The model under review builds one solid part; all positions refer to its coordinate system, in mm. A direction names the side the tool comes from. Coordinates: 2 decimals unless noted, no trailing zeros. Loops run counter-clockwise (first coordinate to the right, second up) from the corner with the lowest first, then second, coordinate; pieces in that order, holes last. Notation, with made-up numbers: M 52.25,75 L 64.25,75 A13 cw 64.25,79 Z; hole C -31,-33.5 d8. An arc over 180 degrees is marked long. Return JSON: item names as keys, results as strings.
```python
from build123d import *

# Parameters (mm, degrees)
F0_R     = 200
F0_R_2   = 198
F1_DEPTH = 655
F0_R_3   = 240
F0_R_4   = 6
F2_DEPTH = 5
F4_R     = 5
F5_SIZE  = 1
F6_SIZE  = 1
F8_D     = 300
F8_DEPTH = 240.001


# Not quite as in the source:
# - a fillet or chamfer that OpenCascade refuses, or shapes differently, is made with other operations: its cross-section is extruded or revolved along the edge and cut away or added
# - a feature names something its author has since deleted; it is built from what else it names


with BuildPart() as f1:
    # F0 (on Front) → F1 (new body)
    with BuildSketch(Plane.XZ):
        Circle(F0_R)
        Circle(F0_R_2, mode=Mode.SUBTRACT)
    extrude(amount=F1_DEPTH)

    # F0 (on Front) → F2 (join)
    with BuildSketch(Plane.XZ):
        Circle(F0_R_3)
        with Locations((-148.3494010818, -162.4575489125)):
            Circle(F0_R_4, mode=Mode.SUBTRACT)
        with Locations((-24.5270352061, -218.6285080771)):
            Circle(F0_R_4, mode=Mode.SUBTRACT)
        with Locations((-215.5073379549, -44.2333277925)):
            Circle(F0_R_4, mode=Mode.SUBTRACT)
        with Locations((108.663824475, -191.2908080658)):
            Circle(F0_R_4, mode=Mode.SUBTRACT)
        with Locations((200.3487965542, -90.8865211088)):
            Circle(F0_R_4, mode=Mode.SUBTRACT)
        with Locations((-200.0304758549, 90.5413627625)):
            Circle(F0_R_4, mode=Mode.SUBTRACT)
        with Locations((-108.663824475, 191.2908080658)):
            Circle(F0_R_4, mode=Mode.SUBTRACT)
        Circle(F0_R, mode=Mode.SUBTRACT)
        with Locations((215.5073379549, 44.2333277925)):
            Circle(F0_R_4, mode=Mode.SUBTRACT)
        with Locations((23.8151364028, 219.3368971348)):
            Circle(F0_R_4, mode=Mode.SUBTRACT)
        with Locations((148.3494010818, 162.4575489125)):
            Circle(F0_R_4, mode=Mode.SUBTRACT)
        Circle(F0_R)
        Circle(F0_R_2, mode=Mode.SUBTRACT)
    extrude(amount=-F2_DEPTH)

    # F3: fillet of radius 5 on 1 edges, made by hand

    # F3_s1 → F3_t2 (revolve, cut)
    with BuildSketch(Plane.XY):
        with BuildLine():
            ThreePointArc((198, 0), (199.4644660941, 3.5355339059), (203, 5))
            Line((203, 5), (198, 5))
            Line((198, 5), (198, 0))
        make_face()
    revolve(axis=Axis((0, 5, 0), (0, -1, 0)), mode=Mode.SUBTRACT)

    # F4
    f4_edges = [f1.edges().sort_by_distance(p)[0] for p in [
        (-200, 0, 0),
    ]]
    fillet(f4_edges, radius=F4_R)

    # F5
    f5_edges = [f1.edges().sort_by_distance(p)[0] for p in [
        (-205, 0, 0),
        (-240, 0, 0),
        (-154.349401, 0, -162.457549),
        (-30.527035, 0, -218.628508),
        (-221.507338, 0, -44.233328),
        (102.663824, 0, -191.290808),
        (194.348797, 0, -90.886521),
        (-206.030476, 0, 90.541363),
        (-114.663824, 0, 191.290808),
        (209.507338, 0, 44.233328),
        (17.815136, 0, 219.336897),
        (142.349401, 0, 162.457549),
    ]]
    chamfer(f5_edges, length=F5_SIZE)

    # F6
    f6_edges = [f1.edges().sort_by_distance(p)[0] for p in [
        (-240, 5, 0),
        (-154.349401, 5, -162.457549),
        (-30.527035, 5, -218.628508),
        (-221.507338, 5, -44.233328),
        (102.663824, 5, -191.290808),
        (-203, 5, 0),
        (194.348797, 5, -90.886521),
        (-206.030476, 5, 90.541363),
        (-114.663824, 5, 191.290808),
        (209.507338, 5, 44.233328),
        (17.815136, 5, 219.336897),
        (142.349401, 5, 162.457549),
    ]]
    chamfer(f6_edges, length=F6_SIZE)

    # F8 (through all, one way)
    with BuildSketch(Plane(origin=(0, 0, 0), x_dir=(1, 0, 0), z_dir=(0, 0, -1))):
        with Locations((0, 178.1619042158)):
            Circle(F8_D / 2)
    extrude(amount=-F8_DEPTH, mode=Mode.SUBTRACT)


solid = f1.part
```
1. The part is to be moulded in two halves that separate along Y. For faces 3 (the face through (104.52, -285.75, 169.7)), 4 (the face through (-239.77, 2.48, 10.55)), 5 (the face through (-54, 5, 196)), 6 (the face through (194, 0, 72)), say which applies: released by +Y, released by -Y, zero draft, split by the parting line, or undercut.
Check values:
{"face 3": "undercut", "face 4": "zero draft", "face 5": "released by +Y", "face 6": "released by -Y"}
2. Add section B-B on z = 0. Give the boundary of the cut face in (x, y).
Check values:
{"outline": "M -240,1 L -239,0 L -205,0 A5 cw -200,-5 L -200,-655 L -198,-655 L -198,0 A5 ccw -203,5 L -239,5 L -240,4 Z; M 198,-655 L 200,-655 L 200,-5 A5 cw 205,0 L 239,0 L 240,1 L 240,4 L 239,5 L 203,5 A5 ccw 198,0 Z"}
3. Add section C-C on y = -349. Give the boundary of the cut face in (x, z).
Check values:
{"outline": "C 0,0 d400; hole C 0,0 d396"}
4. Insertion check: pin 1 Ø11 at (x, z) = (108.66, -191.29) entering from -Y; pin 2 Ø19 at (x, z) = (-215.51, -44.23) entering from -Y; pin 3 Ø8 at (x, y) = (94, -250) entering from +Z; pin 4 Ø1 at (y, z) = (-350, -75) entering from -X. Each pin has a flat end and moves straight along its axis. Give the tip position at first contact, or say it passes through.
Check values:
{"pin 1": "through", "pin 2": "y = 0", "pin 3": "z = -172.05", "pin 4": "x = -185.61"}
5. Add section D-D on y = -189. Give the boundary of the cut face in (x, z).
Check values:
{"outline": "M -149.61,129.7 L -149.61,132.73 A200 ccw long 149.61,132.73 L 149.61,129.7 A198 cw long Z"}
6. Machinability: for faces 1 (the face through (-194, -655, 45)), 2 (the face through (-43.356, -325.45, -195.244)), which of the approach directions +Z, -Z, +X, -X, +Y, -Y give a long, thin tool a straight path to every point of the face, cutting with its end or side? Answer none if there is none.
Check values:
{"face 1": "+Z, -Z, +X, -X, -Y", "face 2": "-Y"}
7. To check wall thickness, follow line 1 (X direction, y = -199, z = -3); line 2 (Z direction, x = 8.5, y = -376); line 3 (Y direction, x = -133.5, z = -176). State the ranges of each line that lie inside material, in increasing order.
Check values:
{"line 1": "-199.98 to -197.98, 197.98 to 199.98", "line 2": "-199.82 to -197.82, 197.82 to 199.82", "line 3": "0 to 5"}
8. Add section A-A on x = 0. Give the boundary of the cut face in (y, z), plus the area to 3 significant figures.
Check values:
{"outline": "M -655,-200 L -5,-200 A5 cw 0,-205 L 0,-239 L 1,-240 L 4,-240 L 5,-239 L 5,-203 A5 ccw 0,-198 L -655,-198 Z; M -655,198 L -328.16,198 L -328.16,200 L -655,200 Z; M -28.16,198 L 0,198 A5 ccw 5,203 L 5,239 L 4,240 L 1,240 L 0,239 L 0,205 A5 cw -5,200 L -28.16,200 Z", "area": "2,440 mm²"}
